Drawing for the job (mm, zero at the part's lowest x, y, z). Coordinates: 2 decimals unless noted, no trailing zeros. Loops run counter-clockwise (first coordinate to the right, second up) from the corner with the lowest first, then second, coordinate; pieces in that order, holes last. Notation, with made-up numbers: (46, 60) -> (81, 60) arc R21 ccw to (81, 69) -> close; hole circle Ø6 at (70, 39). An arc over 180 degrees is marked (long way). Write item = value, one per line. Start each with the question number.
(1) Drill centre lines: line 1 (Z direction, x = 8.5, y = 7.25) (1 decimal); line 2 (X direction, y = 1, z = 15.25) (1 decimal); line 3 (Z direction, x = 5.5, y = 8.75) (1 decimal). Where is each one in solid material? Low to high. Write a range as from..to.
(2) Flat gauge pins, fed straight in: P1, Ø1, axis at x = 3, z = 11.5, coming from the +Y side; P2, Ø4, axis at y = 1.5, z = 21, coming from the -X side (1 decimal); P3, Ø8, axis at x = 2, z = 5.5, coming from the -Y side (1 decimal). Where does each tip first touch, or does it go through?
(3) Band-saw the part on B-B (z = 14). Write the cut outline in (x, y) (1 decimal).
(4) Pull direction Z, two halves, no side cores. Call the marked faces 1, 2, 3 and 4: +Z half, -Z half, draft (parallel to the pull), parting line (faces both ways), or undercut.
(5) Band-saw the part on A-A (x = 8.5). Write the cut outline in (y, z) (1 decimal).
(6) Band-saw the part on D-D (z = 20.5). Write the cut outline in (x, y).
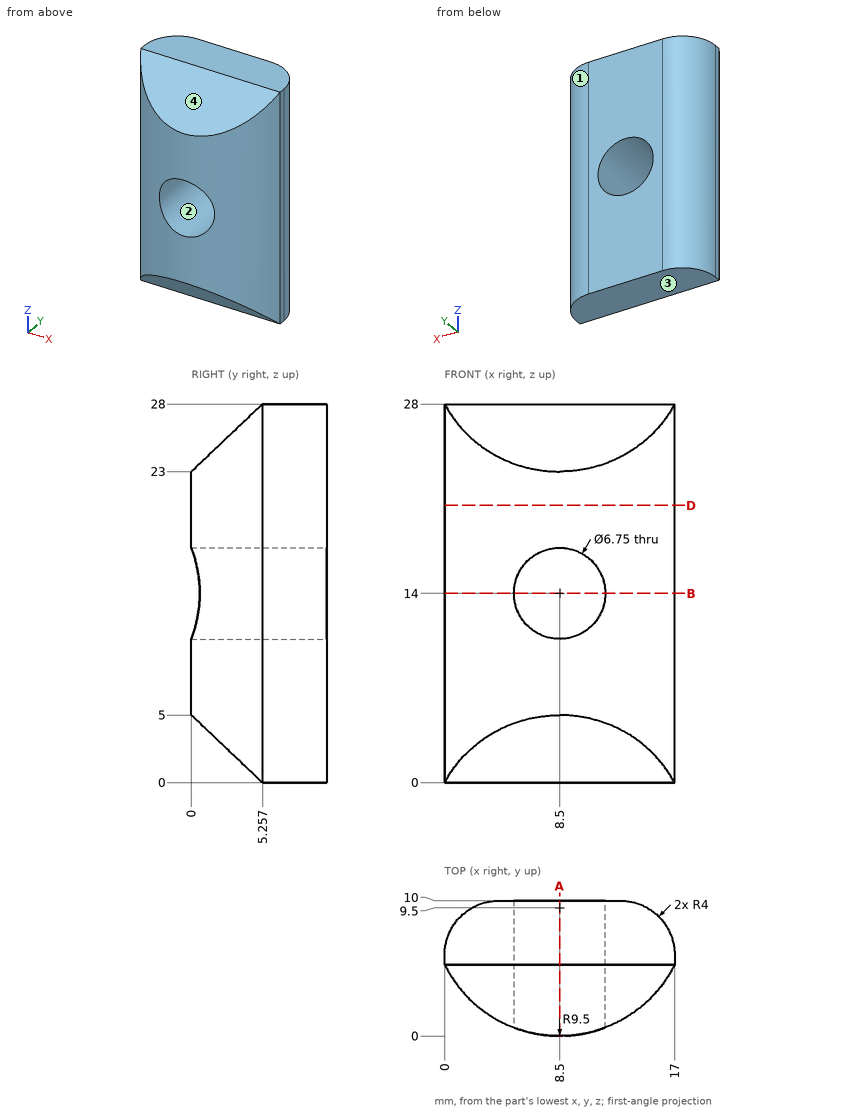
Findings below:
q1.line_1 = 0..10.6, 17.4..28
q1.line_2 = 4.3..5.4, 11.6..12.7
q1.line_3 = 0..12.5, 15.5..28
q2.P1 = 9.97
q2.P2 = 1.1
q2.P3 = 0.3
q3.outline = (0, 5.3) arc R9.5 ccw to (5.1, 0.6) -> (5.1, 10) -> (4, 10) arc R4 ccw to (0, 6) -> close; (11.9, 0.6) arc R9.5 ccw to (17, 5.3) -> (17, 6) arc R4 ccw to (13, 10) -> (11.9, 10) -> close
q4.face_1 = draft
q4.face_2 = undercut
q4.face_3 = -Z half
q4.face_4 = +Z half
q5.outline = (0, 5) -> (5.3, 0) -> (10, 0) -> (10, 10.6) -> (0, 10.6) -> close; (0, 17.4) -> (10, 17.4) -> (10, 28) -> (5.3, 28) -> (0, 23) -> close
q6.outline = (0, 5.26) arc R9.5 ccw to (17, 5.26) -> (17, 6) arc R4 ccw to (13, 10) -> (4, 10) arc R4 ccw to (0, 6) -> close
